```python
from build123d import *

# Parameters (mm, degrees)
F0_R     = 10
F1_DEPTH = 10
F3_DEPTH = 5
F5_DEPTH = 40
F6_SIZE  = 1
F8_DEPTH = 16


with BuildPart() as f1:
    # F0 (on Top) → F1 (new body)
    with BuildSketch(Plane.XY):
        with BuildLine():
            Line((-20, 120), (-20, 0))
            ThreePointArc((-20, 0), (-14.96663, -13.266499), (-2.4, -19.855478))
            ThreePointArc((-2.4, -19.855478), (0.741657, -21.502723), (2, -24.819347))
            Line((2, -24.819347), (2, -120))
            ThreePointArc((2, -120), (3.464466, -123.535534), (7, -125))
            Line((7, -125), (15, -125))
            ThreePointArc((15, -125), (18.535534, -123.535534), (20, -120))
            Line((20, -120), (20, 0))
            ThreePointArc((20, 0), (14.96663, 13.266499), (2.4, 19.855478))
            ThreePointArc((2.4, 19.855478), (-0.741657, 21.502723), (-2, 24.819347))
            Line((-2, 24.819347), (-2, 81.492189))
            ThreePointArc((-2, 81.492189), (-1.436283, 84.802259), (0.191312, 87.73914))
            Line((0.191312, 87.73914), (1.500244, 89.375305))
            ThreePointArc((1.500244, 89.375305), (1.719375, 90), (1.500244, 90.624695))
            Line((1.500244, 90.624695), (0.191312, 92.26086))
            ThreePointArc((0.191312, 92.26086), (-1.436283, 95.197741), (-2, 98.507811))
            Line((-2, 98.507811), (-2, 120))
            ThreePointArc((-2, 120), (-3.464466, 123.535534), (-7, 125))
            Line((-7, 125), (-15, 125))
            ThreePointArc((-15, 125), (-18.535534, 123.535534), (-20, 120))
        make_face()
        Circle(F0_R, mode=Mode.SUBTRACT)
    extrude(amount=F1_DEPTH)

    # F2 (on face) → F3 (cut)
    with BuildSketch(Plane.XY.offset(10)):
        with BuildLine():
            Line((12.204651, -20), (20, -20))
            Line((20, -20), (20, 25))
            Line((20, 25), (-2, 25))
            Line((-2, 25), (-6.392269, 21.862665))
            ThreePointArc((-6.392269, 21.862665), (-9.152876, 20.477045), (-12.204651, 20))
            Line((-12.204651, 20), (-20, 20))
            Line((-20, 20), (-20, -25))
            Line((-20, -25), (2, -25))
            Line((2, -25), (6.392269, -21.862665))
            ThreePointArc((6.392269, -21.862665), (9.152876, -20.477045), (12.204651, -20))
        make_face()
    extrude(amount=-F3_DEPTH, mode=Mode.SUBTRACT)

    # F4 (on face) → F5 (join)
    with BuildSketch(Plane.XY.offset(10)):
        with BuildLine():
            Line((-7, 125), (-15, 125))
            ThreePointArc((-15, 125), (-18.535534, 123.535534), (-20, 120))
            Line((-20, 120), (-20, 118))
            ThreePointArc((-20, 118), (-17.656854, 112.343146), (-12, 110))
            Line((-12, 110), (-10, 110))
            ThreePointArc((-10, 110), (-4.343146, 112.343146), (-2, 118))
            Line((-2, 118), (-2, 120))
            ThreePointArc((-2, 120), (-3.464466, 123.535534), (-7, 125))
        make_face()
        with BuildLine():
            Line((7, -125), (15, -125))
            ThreePointArc((15, -125), (18.535534, -123.535534), (20, -120))
            Line((20, -120), (20, -118))
            ThreePointArc((20, -118), (17.656854, -112.343146), (12, -110))
            Line((12, -110), (10, -110))
            ThreePointArc((10, -110), (4.343146, -112.343146), (2, -118))
            Line((2, -118), (2, -120))
            ThreePointArc((2, -120), (3.464466, -123.535534), (7, -125))
        make_face()
    extrude(amount=F5_DEPTH)

    # F6
    f6_edges = [f1.edges().sort_by_distance(p)[0] for p in [
        (-10, 0, 0),
    ]]
    chamfer(f6_edges, length=F6_SIZE)

    # F7 (on face) → F8 (cut)
    with BuildSketch(Plane(origin=(0, 0, 0), x_dir=(1, 0, 0), z_dir=(0, 0, -1))):
        with BuildLine():
            Line((13.65, 120.65), (8.35, 120.65))
            ThreePointArc((8.35, 120.65), (6.935786, 120.064214), (6.35, 118.65))
            Line((6.35, 118.65), (6.35, 116.35))
            ThreePointArc((6.35, 116.35), (6.935786, 114.935786), (8.35, 114.35))
            Line((8.35, 114.35), (13.65, 114.35))
            ThreePointArc((13.65, 114.35), (15.064214, 114.935786), (15.65, 116.35))
            Line((15.65, 116.35), (15.65, 118.65))
            ThreePointArc((15.65, 118.65), (15.064214, 120.064214), (13.65, 120.65))
        make_face()
        with BuildLine():
            Line((-8.35, -114.35), (-13.65, -114.35))
            ThreePointArc((-13.65, -114.35), (-15.064214, -114.935786), (-15.65, -116.35))
            Line((-15.65, -116.35), (-15.65, -118.65))
            ThreePointArc((-15.65, -118.65), (-15.064214, -120.064214), (-13.65, -120.65))
            Line((-13.65, -120.65), (-8.35, -120.65))
            ThreePointArc((-8.35, -120.65), (-6.935786, -120.064214), (-6.35, -118.65))
            Line((-6.35, -118.65), (-6.35, -116.35))
            ThreePointArc((-6.35, -116.35), (-6.935786, -114.935786), (-8.35, -114.35))
        make_face()
    extrude(amount=-F8_DEPTH, mode=Mode.SUBTRACT)


solid = f1.part
```
The model under review builds one solid part; all positions refer to its coordinate system, in mm. A direction names the side the tool comes from. Give positions to 0.01 mm unless a question says otherwise; leave off trailing zeros. Loops run counter-clockwise (first coordinate to the right, second up) from the corner with the lowest first, then second, coordinate; pieces in that order, holes last. Notation, with made-up numbers: (2, 66.5) - (31, 66.5) arc R21 cw to (31, 81.5) - close; hole circle Ø7 at (3, 89). An arc over 180 degrees is marked (long way). Answer as a JSON object with one key per item and string values.
Q1. Add section B-B on y = -33. State the section outline as (x, z) points.
Worked out:
{"outline": "(2, 0) - (20, 0) - (20, 10) - (2, 10) - close"}
Q2. Insertion check: pin 1 (24 mm diameter, centred on x = -13.5, y = 48, fed in from +Z); pin 2 (8 mm diameter, centred on x = -10, y = -23.5, fed in from +Z); pin 3 (4 mm diameter, centred on x = 7, z = 19, fed in from +Y); pin 4 (4 mm diameter, centred on x = 17, z = 8, fed in from +Y). Each pin has a flat end and moves straight along its axis. Give the tip position at first contact, or say it passes through.
Worked out:
{"pin 1": "stops at z = 10", "pin 2": "passes through", "pin 3": "stops at y = -110.06", "pin 4": "stops at y = -20"}
Q3. To check wall thickness, follow line 1 along Y through (x, z) = (-11.5, 9.5); line 2 along Z through (x, y) = (14, -60); line 3 along Y through (x, z) = (0, 2.35). State the ranges of each line that lie inside material, in increasing order.
Worked out:
{"line 1": "y = 20.02 to 114.35, 120.65 to 125", "line 2": "z = 0 to 10", "line 3": "y = -20.82 to -10, 10 to 20.82, 87.49 to 92.51"}
Q4. Add section A-A on z = 30. State the section outline as (x, y) points.
Worked out:
{"outline": "(-20, 118) arc R8 ccw to (-12, 110) - (-10, 110) arc R8 ccw to (-2, 118) - (-2, 120) arc R5 ccw to (-7, 125) - (-15, 125) arc R5 ccw to (-20, 120) - close; (2, -120) arc R5 ccw to (7, -125) - (15, -125) arc R5 ccw to (20, -120) - (20, -118) arc R8 ccw to (12, -110) - (10, -110) arc R8 ccw to (2, -118) - close"}
Q5. For faces 4 (the cylindrical face through (-4.406, 112.281, 29.72)), 5 (the cylindrical face through (17.719, -112.406, 29.72)), 6 (the cylindrical face through (-17.719, 112.406, 29.72)), 7 (the flat face through (-11, 114.35, 8)), list the 3-axis set-ups (+Z, -Z, +X, -X, +Y, -Y) from which the entire face can be reached by the end or side of a thin tool; tool diameter is ignored.
Worked out:
{"face 4": "+Z, +X, -Y", "face 5": "+Z, +X, +Y", "face 6": "+Z, -X, -Y", "face 7": "-Z"}
Q6. Mouldability with a two-part tool opening along Y and no side actions: class faces 1 (the flat face through (4.17, -23.45, 7.54)), 2 (the flat face through (11, -117, 50)), 3 (the cylindrical face through (-1.45, 84.76, 4.93)) as +Y half, -Y half, draft (parallel to the pull), parting line (faces both ways), or undercut.
Worked out:
{"face 1": "+Y half", "face 2": "draft", "face 3": "undercut"}
